Input: part model. Units: mm. Frame: model coordinates. Coordinates: 2 decimals unless noted, no trailing zeros. Order: outer loops, then holes, each group sorted by start corner. A loop starts at its lowest first (then second) coordinate and runs counter-clockwise, first axis right, second up.
from build123d import *

# Parameters (mm, degrees)
SKETCH_1_W           = 0.64
SKETCH_1_H           = 0.64
EXTRUDE_1_DEPTH      = 2.54
SKETCH_1_2_W         = 0.64
SKETCH_1_2_H         = 0.64
EXTRUDE_2_DEPTH      = 5.3
EXTRUDE_2_DEPTH_BACK = 6


with BuildPart() as part:
    # Sketch 1 → Extrude 1 (new body)
    with BuildSketch(Plane(origin=(0, 0, 0), x_dir=(1, 0, 0), z_dir=(0, 1, 0))):
        with BuildLine():
            Line((0.97, -1.27), (-0.97, -1.27))
            ThreePointArc((-0.97, -1.27), (-1.182132034, -1.182132034), (-1.27, -0.97))
            Line((-1.27, -0.97), (-1.27, 0.97))
            ThreePointArc((-1.27, 0.97), (-1.182132034, 1.182132034), (-0.97, 1.27))
            Line((-0.97, 1.27), (0.97, 1.27))
            ThreePointArc((0.97, 1.27), (1.182132034, 1.182132034), (1.27, 0.97))
            Line((1.27, 0.97), (1.27, -0.97))
            ThreePointArc((1.27, -0.97), (1.182132034, -1.182132034), (0.97, -1.27))
        make_face()
        Rectangle(SKETCH_1_W, SKETCH_1_H, mode=Mode.SUBTRACT)
    extrude(amount=EXTRUDE_1_DEPTH)

    # Sketch 1_2 → Extrude 2 (add, two sides)
    with BuildSketch(Plane(origin=(0, 0, 0), x_dir=(1, 0, 0), z_dir=(0, 1, 0))) as extrude_2_sk:
        Rectangle(SKETCH_1_2_W, SKETCH_1_2_H)
    extrude(amount=EXTRUDE_2_DEPTH)
    extrude(extrude_2_sk.sketch, amount=-EXTRUDE_2_DEPTH_BACK)


solid = part.part
Item 1: Ray query, probe 1 along Y at (x, z) = (-0.1, 0.75); probe 2 along Z at (x, y) = (0.15, 4.5). Return the intervals inside material, ascending.
Response values:
probe 1: y = 0 to 2.54
probe 2: z = -0.32 to 0.32
Item 2: Cut plane B-B on z = -0.7. Return loops of the section in (x, y).
Response values:
outline: (-1.27, 0) - (1.27, 0) - (1.27, 2.54) - (-1.27, 2.54) - close
Item 3: Cut plane C-C on y = -4. Return loops of the section in (x, z), then the cut area to 3 significant figures.
Response values:
outline: (-0.32, -0.32) - (0.32, -0.32) - (0.32, 0.32) - (-0.32, 0.32) - close
area: 0.410 mm2
Item 4: Pin query (flat end, axial travel): pin 1 Ø1 at (y, z) = (-1, 0) entering from +X; pin 2 Ø0.7 at (x, y) = (0, -3.5) entering from +Z; pin 3 Ø0.5 at (y, z) = (-4.5, 0) entering from -X. Return the tip coordinate at first contact, or that it passes through.
Response values:
pin 1: stops at x = 0.32
pin 2: stops at z = 0.32
pin 3: stops at x = -0.32
Item 5: Cut plane A-A on x = 0.05. Return loops of the section in (y, z), then the cut area to 3 significant figures.
Response values:
outline: (-6, -0.32) - (0, -0.32) - (0, -1.27) - (2.54, -1.27) - (2.54, -0.32) - (5.3, -0.32) - (5.3, 0.32) - (2.54, 0.32) - (2.54, 1.27) - (0, 1.27) - (0, 0.32) - (-6, 0.32) - close
area: 12.1 mm2
